The model under review builds one solid part; all positions refer to its coordinate system, in mm. Coordinates: 2 decimals unless noted, no trailing zeros. Loops run counter-clockwise (first coordinate to the right, second up) from the corner with the lowest first, then second, coordinate; pieces in that order, holes last. Notation, with made-up numbers: (11, 41) - (66, 41) arc R15 ccw to (66, 53) - close; hole circle Ø8 at (29, -29.5). An arc over 180 degrees is marked (long way). Answer in a Markdown table with one row per item. Add a question column.
(1) We need section D-D on y = -333. Write out the cut boundary in (x, z).
(2) We need section A-A on y = -739.81. Write out the cut boundary in (x, z), plus the area to 3 significant figures.
(3) We need section B-B on y = -1153.86. Write out the cut boundary in (x, z).
(4) For P1, Ø8, axis at x = -495.5, y = -821.5, coming from the -Z side; P2, Ø1.5, axis at y = -640.5, z = 8, coming from the +X side; P3, Ø3.5, axis at y = -674, z = 7, coming from the -X side; P4, Ø23, axis at x = -451.35, y = -361.92, coming from the +Z side, all flat-tipped, find the tip position at first contact; note any pin that passes through.
(5) We need section C-C on z = 7. Give the number of separate pieces and of enclosed holes in the cut face, plus the area to 3 significant figures.
(6) For line 1 along X through (y, z) = (-600.29, 13); line 2 along X through (y, z) = (-228.93, 7.5); line 3 along Y through (x, z) = (-45.58, 4.75), list the stretches that pass through material, from the lowest coordinate up.
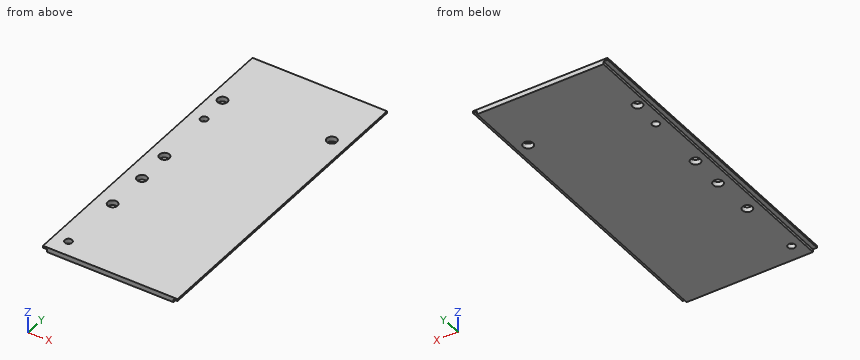
from build123d import *

# Parameters (mm, degrees)
SKETCH1_W           = 488.95
SKETCH1_H           = 1219.2
SKETCH1_R           = 14.035
SKETCH1_R_2         = 19.005
SKETCH1_R_3         = 19.085
SKETCH1_R_4         = 19.265
SKETCH1_R_5         = 14.26
SKETCH1_R_6         = 19.135
SKETCH1_R_7         = 19.38
SKETCH1_W_2         = 15.83
BOSS_EXTRUDE1_DEPTH = 19.05
SKETCH1_3_W         = 15.83
SKETCH1_3_H         = 1219.2
CUT_EXTRUDE1_DEPTH  = 11.05


with BuildPart() as part:
    # Sketch1 → Boss-Extrude1 (new body)
    # profile 1 of 3: a face of its own
    with BuildSketch(Plane.XY):
        with Locations((-244.475, -609.6)):
            Rectangle(SKETCH1_W, SKETCH1_H)
        with Locations(Location((-449.645, -1153.86, 0), (0, 0, 180))):
            Circle(SKETCH1_R, mode=Mode.SUBTRACT)
        with Locations(Location((-443.355, -906.4175, 0), (0, 0, 180))):
            Circle(SKETCH1_R_2, mode=Mode.SUBTRACT)
        with Locations(Location((-440.665, -739.81, 0), (0, 0, 180))):
            Circle(SKETCH1_R_3, mode=Mode.SUBTRACT)
        with Locations(Location((-446.415, -600.29, 0), (0, 0, 180))):
            Circle(SKETCH1_R_4, mode=Mode.SUBTRACT)
        with Locations(Location((-451.35, -361.9225, 0), (0, 0, 180))):
            Circle(SKETCH1_R_5, mode=Mode.SUBTRACT)
        with Locations(Location((-458.365, -244.56, 0), (0, 0, 180))):
            Circle(SKETCH1_R_6, mode=Mode.SUBTRACT)
        with Locations(Location((-45.58, -228.93, 0), (0, 0, 180))):
            Circle(SKETCH1_R_7, mode=Mode.SUBTRACT)
    # profile 2 of 3: a face of its own
    with BuildSketch(Plane.XY):
        with Locations((7.915, -609.6)):
            Rectangle(SKETCH1_W_2, SKETCH1_H)
    # profile 3 of 3: a face of its own
    with BuildSketch(Plane.XY):
        with Locations((-496.865, -609.6)):
            Rectangle(SKETCH1_W_2, SKETCH1_H)
    extrude(amount=BOSS_EXTRUDE1_DEPTH)

    # Sketch1_3 → Cut-Extrude1 (cut)
    with BuildSketch(Plane.XY):
        with Locations((-496.865, -609.6)):
            Rectangle(SKETCH1_3_W, SKETCH1_3_H)
        with Locations((7.915, -609.6)):
            Rectangle(SKETCH1_3_W, SKETCH1_3_H)
    extrude(amount=CUT_EXTRUDE1_DEPTH, mode=Mode.SUBTRACT)


solid = part.part
Outcome:
| question | item | result |
|---|---|---|
| 1 | outline | (-504.78, 11.05) - (-488.95, 11.05) - (-488.95, 0) - (0, 0) - (0, 11.05) - (15.83, 11.05) - (15.83, 19.05) - (-504.78, 19.05) - close |
| 2 | outline | (-504.78, 11.05) - (-488.95, 11.05) - (-488.95, 0) - (-459.75, 0) - (-459.75, 19.05) - (-504.78, 19.05) - close; (-421.58, 0) - (0, 0) - (0, 11.05) - (15.83, 11.05) - (15.83, 19.05) - (-421.58, 19.05) - close |
| 2 | area | 8,840 mm² |
| 3 | outline | (-504.78, 11.05) - (-488.95, 11.05) - (-488.95, 0) - (-463.68, 0) - (-463.68, 19.05) - (-504.78, 19.05) - close; (-435.61, 0) - (0, 0) - (0, 11.05) - (15.83, 11.05) - (15.83, 19.05) - (-435.61, 19.05) - close |
| 4 | P1 | z = 11.05 |
| 4 | P2 | x = 0 |
| 4 | P3 | x = -488.95 |
| 4 | P4 | through |
| 5 | separate pieces | 1 |
| 5 | enclosed holes | 7 |
| 5 | area | 589,000 mm² |
| 6 | line 1 | -504.78 to -465.68, -427.15 to 15.83 |
| 6 | line 2 | -488.95 to -469.4, -447.33 to -64.96, -26.2 to 0 |
| 6 | line 3 | -1219.2 to -248.31, -209.55 to 0 |
